Could you check a few things on this model? Use its own coordinates, in mm. A direction names the side the tool comes from. Give positions to 0.01 mm unless a question says otherwise; leave off trailing zeros. Order: outer loops, then holes, each group sorted by start corner. A loop starts at its lowest first (then second) coordinate and runs counter-clockwise, first axis right, second up.
from build123d import *

# Parameters (mm, degrees)
F1_DEPTH = 3.175


# Not quite as in the source:
# - ends of sketch curves that miss each other by under 0.0002 mm in the source are joined


with BuildPart() as f1:
    # F0 (on Front) → F1 (new body)
    with BuildSketch(Plane.XZ):
        Polygon((0, -50.8), (0, 0), (-304.8, -6.031e-07), (-355.6, -101.6), (-256.2067782821, -101.6), (-230.8067781314, -50.8), align=None)
        Polygon((304.8, 0), (0, -3.015e-07), (0, -50.8), (230.8067784001, -50.8), (256.2067784001, -101.6), (355.6, -101.6), align=None)
    extrude(amount=F1_DEPTH)


solid = f1.part
Item 1: Imagine slicing it at C-C on x = -23. List the corners of the cut face in (y, z) for me (3 decimals).
Findings:
outline: (-3.175, -50.8) - (0, -50.8) - (0, 0) - (-3.175, 0) - close
Item 2: We'd pull the mould along X, two halves only. Please class faces 3 (the flat face through (-5, 0, -39)), 4 (the flat face through (330.556, -1.565, -51.511)), 5 (the flat face through (-243.685, -1.565, -76.556)), 6 (the flat face through (-329.844, -1.565, -50.089)): +X half, -X half, draft (parallel to the pull), parting line (faces both ways), or undercut.
Findings:
face 3: draft
face 4: +X half
face 5: undercut
face 6: -X half
Item 3: Imagine slicing it at D-D on z = -44.5. List the corners of the cut face in (x, y) for me (3 decimals), then the cut area to 3 significant figures.
Findings:
outline: (-327.05, -3.175) - (327.05, -3.175) - (327.05, 0) - (-327.05, 0) - close
area: 2,080 mm2
Item 4: Please list where these lines run through material, in increasing order: line 1 along Z through (x, y) = (-5, -1.4); line 2 along X through (y, z) = (-0.3, -54); line 3 along X through (y, z) = (-0.55, -93.5).
Findings:
line 1: z = -50.8 to 0
line 2: x = -331.8 to -232.41, 232.41 to 331.8
line 3: x = -351.55 to -252.16, 252.16 to 351.55
Item 5: Imagine slicing it at B-B on z = -91. List the corners of the cut face in (x, y) for me (3 decimals), then the cut area to 3 significant figures.
Findings:
outline: (-350.3, -3.175) - (-250.907, -3.175) - (-250.907, 0) - (-350.3, 0) - close; (250.907, -3.175) - (350.3, -3.175) - (350.3, 0) - (250.907, 0) - close
area: 631 mm2
Item 6: For pin 1 (1.6 mm diameter, centred on x = 7.5, y = -1.5, fed in from -Z); pin 2 (1.5 mm diameter, centred on y = -0.5, z = -48.5, fed in from +X) (3 decimals), each with a flat end and sliding along its axis, tell me the tip position at first contact or that it passes through.
Findings:
pin 1: stops at z = -50.8
pin 2: stops at x = 329.425
Item 7: For faces 1 (the flat face through (-5, -3.175, -39)), 2 (the flat face through (243.329, -1.565, -75.844)), which set-ups out of +Z, -Z, +X, -X, +Y, -Y let a thin tool reach every point of the face, with its end or its side?
Findings:
face 1: +Z, -Z, +X, -X, -Y
face 2: -Z, +Y, -Y
Item 8: Imagine slicing it at A-A on y = -1.7. List the corners of the cut face in (x, z) for me, then the cut area to 3 significant figures.
Findings:
outline: (-355.6, -101.6) - (-256.21, -101.6) - (-230.81, -50.8) - (230.81, -50.8) - (256.21, -101.6) - (355.6, -101.6) - (304.8, 0) - (-304.8, 0) - close
area: 42,400 mm2
